Work out the finished part from the listing and answer in its coordinate system (mm). A direction names the side the tool comes from. Coordinates: 2 decimals unless noted, no trailing zeros. Order: outer loops, then holes, each group sorted by start corner. A loop starts at its lowest first (then second) coordinate and runs counter-clockwise, first axis right, second up. Notation, with made-up numbers: (21, -18.5) -> (26, -18.5) arc R14 cw to (26, 5.5) -> close; hole circle Ø4 at (-39, 13). An arc over 180 degrees is marked (long way). Answer as CSV lines item,"result". Start each with the question number.
Item 1: Each of these flat-tipped pins is pushed along its axis until it touches: pin 1 Ø8 at (x, y) = (-23.57, 4.63) entering from -Z; pin 2 Ø8 at (x, z) = (-35, 10) entering from -Y; pin 3 Ø4.5 at (x, y) = (-23.57, 51.77) entering from -Z; pin 4 Ø7.5 at (x, z) = (9.5, 10.5) entering from -Y. Where does it stop, or does it pass through?
Item 2: Which of the six approach directions +Z, -Z, +X, -X, +Y, -Y give full straight-line access (tool end or side, diameter ignored) to faces 1 (the face through (-1, 152, 20)), 2 (the face through (37.867, 13.309, 11.828)), 3 (the face through (15.12, 16.61, 15.79)), 4 (the face through (-50, 144, 10)), 5 (the face through (0, 56.4, 7))?
Item 3: Section A-A (y = 213) is taken. Write down the section's boundary in (x, z).
Item 4: For a pull along Z with two mould halves and no side action, classify faces 6 (the face through (34.48, 27.94, 9.73)), 7 (the face through (-1, 100, 10)), 8 (the face through (-21.072, 4.74, 17.465)) as pulls with the +Z half, pulls with the -Z half, needs draft (parallel to the pull), parting line crosses it, or undercut.
Item 5: Straight lines are drawn through the part: L1, parallel to X at y = 12.75, z = 10; L2, parallel to Y at x = -34.5, z = 8.5; L3, parallel to Y at x = -23.57, z = 16.4. For each, find the intervals that lie inside material, in ascending order.
```python
from build123d import *

# Parameters (mm, degrees)
DODANIE_WYCI_GNI_CIE1_DEPTH = 20
DODANIE_WYCI_GNI_CIE2_DEPTH = 5
OTW_R_GWINTOWANY_M81_D      = 6.8
OTW_R_GWINTOWANY_M81_DEPTH  = 26.25
OTW_R_GWINTOWANY_M81_TIP    = 2.042926105
SZKIC4_R                    = 19.05
SZKIC4_R_2                  = 3.25
WYTNIJ_WYCI_GNI_CIE2_DEPTH  = 15
SZKIC4_4_R                  = 19.05
SZKIC4_4_R_2                = 3.25
WYTNIJ_WYCI_GNI_CIE3_DEPTH  = 16.6
SZKIC4_5_R                  = 3.25
WYTNIJ_WYCI_GNI_CIE4_DEPTH  = 49.6
SZKIC5_R                    = 2.5
WYTNIJ_WYCI_GNI_CIE5_DEPTH  = 7.6
WYTNIJ_WYCI_GNI_CIE6_DEPTH  = 10


with BuildPart() as part:
    # Szkic1 → Dodanie-wyci_gni_cie1 (new body)
    with BuildSketch(Plane.XY):
        with BuildLine():
            Line((-50, 0), (0, 0))
            Line((0, 0), (0, 252.5))
            ThreePointArc((0, 252.5), (-17.5, 270), (0, 287.5))
            Line((0, 287.5), (0, 300))
            Line((0, 300), (-21.900286098, 300))
            Line((-21.900286098, 300), (-50, 283.776622614))
            Line((-50, 283.776622614), (-50, 0))
        make_face()
        with BuildLine():
            Line((0, 252.5), (0, 0))
            Line((0, 0), (50, 0))
            Line((50, 0), (50, 283.776622614))
            Line((50, 283.776622614), (21.900286098, 300))
            Line((21.900286098, 300), (0, 300))
            Line((0, 300), (0, 287.5))
            ThreePointArc((0, 287.5), (12.374368671, 282.374368671), (17.5, 270))
            ThreePointArc((17.5, 270), (12.374368671, 257.625631329), (0, 252.5))
        make_face()
    extrude(amount=DODANIE_WYCI_GNI_CIE1_DEPTH)

    # Szkic1_3 → Dodanie-wyci_gni_cie2 (add)
    with BuildSketch(Plane.XY):
        with BuildLine():
            ThreePointArc((0, 287.5), (-17.5, 270), (0, 252.5))
            Line((0, 252.5), (0, 255))
            ThreePointArc((0, 255), (-15, 270), (0, 285))
            Line((0, 285), (0, 287.5))
        make_face()
        with BuildLine():
            Line((0, 255), (0, 252.5))
            ThreePointArc((0, 252.5), (12.374368671, 257.625631329), (17.5, 270))
            ThreePointArc((17.5, 270), (12.374368671, 282.374368671), (0, 287.5))
            Line((0, 287.5), (0, 285))
            ThreePointArc((0, 285), (10.606601718, 280.606601718), (15, 270))
            ThreePointArc((15, 270), (10.606601718, 259.393398282), (0, 255))
        make_face()
    extrude(amount=DODANIE_WYCI_GNI_CIE2_DEPTH)

    # Otw_r gwintowany M81
    with Locations(Plane(origin=(-35, 0, 10), x_dir=(0, 0, -1), z_dir=(0, -1, 0))):
        with Locations((0, 0), (0, 70)):
            Hole(OTW_R_GWINTOWANY_M81_D / 2, depth=OTW_R_GWINTOWANY_M81_DEPTH)
            with Locations((0, 0, -(OTW_R_GWINTOWANY_M81_DEPTH + OTW_R_GWINTOWANY_M81_TIP / 2))):  # 118° drill point
                Cone(0, OTW_R_GWINTOWANY_M81_D / 2, OTW_R_GWINTOWANY_M81_TIP, mode=Mode.SUBTRACT)

    # Szkic4 → Wytnij-wyci_gni_cie2 (cut)
    # profile 1 of 2: a face of its own
    with BuildSketch(Plane(origin=(0, 0, 0), x_dir=(-1, 0, 0), z_dir=(0, 0, -1))):
        with BuildLine():
            Line((-28.2, 53.4), (-28.2, 0))
            Line((-28.2, 0), (28.2, 0))
            Line((28.2, 0), (28.2, 53.4))
            ThreePointArc((28.2, 53.4), (27.321320344, 55.521320344), (25.2, 56.4))
            Line((25.2, 56.4), (-25.2, 56.4))
            ThreePointArc((-25.2, 56.4), (-27.321320344, 55.521320344), (-28.2, 53.4))
        make_face()
        with Locations((0, 28.2)):
            Circle(SZKIC4_R, mode=Mode.SUBTRACT)
    # profile 2 of 2: a face of its own
    with BuildSketch(Plane(origin=(0, 0, 0), x_dir=(-1, 0, 0), z_dir=(0, 0, -1))):
        with Locations((0, 28.2)):
            Circle(SZKIC4_R)
        with Locations((0, 28.2)):
            Circle(SZKIC4_R_2, mode=Mode.SUBTRACT)
    extrude(amount=-WYTNIJ_WYCI_GNI_CIE2_DEPTH, mode=Mode.SUBTRACT)

    # Szkic4_4 → Wytnij-wyci_gni_cie3 (cut)
    with BuildSketch(Plane(origin=(0, 0, 0), x_dir=(-1, 0, 0), z_dir=(0, 0, -1))):
        with Locations((0, 28.2)):
            Circle(SZKIC4_4_R)
        with Locations((0, 28.2)):
            Circle(SZKIC4_4_R_2, mode=Mode.SUBTRACT)
    extrude(amount=-WYTNIJ_WYCI_GNI_CIE3_DEPTH, mode=Mode.SUBTRACT)

    # Szkic4_5 → Wytnij-wyci_gni_cie4 (cut)
    with BuildSketch(Plane(origin=(0, 0, 0), x_dir=(-1, 0, 0), z_dir=(0, 0, -1))):
        with Locations((0, 28.2)):
            Circle(SZKIC4_5_R)
    extrude(amount=-WYTNIJ_WYCI_GNI_CIE4_DEPTH, mode=Mode.SUBTRACT)

    # Szkic5 → Wytnij-wyci_gni_cie5 (cut)
    with BuildSketch(Plane(origin=(0, 0, 15), x_dir=(-1, 0, 0), z_dir=(0, 0, -1))):
        with Locations((-23.57, 51.77)):
            Circle(SZKIC5_R)
        with Locations((23.57, 51.77)):
            Circle(SZKIC5_R)
        with Locations((23.57, 4.63)):
            Circle(SZKIC5_R)
        with Locations((-23.57, 4.63)):
            Circle(SZKIC5_R)
    extrude(amount=-WYTNIJ_WYCI_GNI_CIE5_DEPTH, mode=Mode.SUBTRACT)

    # Szkic6 → Wytnij-wyci_gni_cie6 (cut)
    with BuildSketch(Plane(origin=(0, 0, 0), x_dir=(-1, 0, 0), z_dir=(0, 0, -1))):
        with BuildLine():
            Line((-45, 228.928061115), (-45, 82.471938885))
            ThreePointArc((-45, 82.471938885), (-43.078190139, 80.039718467), (-40.267443069, 81.346910197))
            Line((-40.267443069, 81.346910197), (-5.067175687, 151.199885246))
            ThreePointArc((-5.067175687, 151.199885246), (-3.997403411, 155.7), (-5.067175687, 160.200114754))
            Line((-5.067175687, 160.200114754), (-40.267443069, 230.053089803))
            ThreePointArc((-40.267443069, 230.053089803), (-43.078190139, 231.360281533), (-45, 228.928061115))
        make_face()
        with BuildLine():
            Line((2.232556931, 145.714200914), (38.342819518, 74.055390936))
            ThreePointArc((38.342819518, 74.055390936), (38.218169264, 71.13215965), (35.663751201, 69.70535651))
            Line((35.663751201, 69.70535651), (-35.663751201, 69.70535651))
            ThreePointArc((-35.663751201, 69.70535651), (-38.218169264, 71.13215965), (-38.342819518, 74.055390936))
            Line((-38.342819518, 74.055390936), (-2.232556931, 145.714200914))
            ThreePointArc((-2.232556931, 145.714200914), (0, 147.089172226), (2.232556931, 145.714200914))
        make_face()
        with BuildLine():
            Line((45, 228.928061115), (45, 82.471938885))
            ThreePointArc((45, 82.471938885), (43.078190139, 80.039718467), (40.267443069, 81.346910197))
            Line((40.267443069, 81.346910197), (5.067175687, 151.199885246))
            ThreePointArc((5.067175687, 151.199885246), (3.997403411, 155.7), (5.067175687, 160.200114754))
            Line((5.067175687, 160.200114754), (40.267443069, 230.053089803))
            ThreePointArc((40.267443069, 230.053089803), (43.078190139, 231.360281533), (45, 228.928061115))
        make_face()
        with BuildLine():
            Line((-40.008452698, 240.649965574), (-2.232556931, 165.685799086))
            ThreePointArc((-2.232556931, 165.685799086), (0, 164.310827774), (2.232556931, 165.685799086))
            Line((2.232556931, 165.685799086), (40.008452698, 240.649965574))
            ThreePointArc((40.008452698, 240.649965574), (39.883802443, 243.57319686), (37.329384381, 245))
            Line((37.329384381, 245), (-37.32938438, 245))
            ThreePointArc((-37.32938438, 245), (-39.883802443, 243.57319686), (-40.008452698, 240.649965574))
        make_face()
    extrude(amount=-WYTNIJ_WYCI_GNI_CIE6_DEPTH, mode=Mode.SUBTRACT)


solid = part.part
```
Checked values:
1,pin 1,"stops at z = 15"
1,pin 2,"stops at y = 0"
1,pin 3,"passes through"
1,pin 4,"stops at y = 56.4"
2,face 1,"+Z, +X, -X, +Y, -Y"
2,face 2,"-Y"
2,face 3,"-Z"
2,face 4,"+Z, -Z, -X, +Y, -Y"
2,face 5,"-Z, -Y"
3,outline,"(-50, 0) -> (-45, 0) -> (-45, 10) -> (-31.67, 10) -> (-31.67, 0) -> (-26.08, 0) -> (-26.08, 10) -> (26.08, 10) -> (26.08, 0) -> (31.67, 0) -> (31.67, 10) -> (45, 10) -> (45, 0) -> (50, 0) -> (50, 20) -> (-50, 20) -> close"
4,face 6,"undercut"
4,face 7,"pulls with the -Z half"
4,face 8,"needs draft"
5,L1,"x = -50 to -38.4, -31.6 to -28.2, 28.2 to 31.6, 38.4 to 50"
5,L2,"y = 27.34 to 69.71, 81.68 to 92.79, 218.61 to 229.72, 245 to 292.73"
5,L3,"y = 0 to 2.13, 7.13 to 49.27, 54.27 to 299.04"
